Could you check a few things on this model? Use its own coordinates, in mm. A direction names the side the tool comes from. Give positions to 0.01 mm unless a question says otherwise; leave off trailing zeros. Loops run counter-clockwise (first coordinate to the right, second up) from the corner with the lowest first, then second, coordinate; pieces in that order, holes last. Notation, with made-up numbers: M 11,44 L 70,44 A14 ccw 70,51 Z; hole C 26,-20.75 d2. An arc over 180 degrees is marked long. Use CSV: the item, a comma, the result in double quotes.
```python
from build123d import *

# Parameters (mm, degrees)
F1_DEPTH = 12.7
F3_DEPTH = 12.7
F4_W     = 12.7
F4_H     = 38.1
F5_DEPTH = 12.7
F6_R     = 6.35
F7_DEPTH = 25.4
F8_R     = 6.34999


# Not quite as in the source:
# - a fillet or chamfer is up to 0.001 mm smaller than in the source, because OpenCascade refuses the exact size


with BuildPart() as f1:
    # F0 (on Top) → F1 (new body)
    with BuildSketch(Plane.XY):
        with BuildLine():
            ThreePointArc((29.6785237075, -38.1), (48.7285237075, -19.05), (29.6785237075, 0))
            Line((29.6785237075, 0), (-21.1214762925, 0))
            Line((-21.1214762925, 0), (-21.1214762925, -38.1))
            Line((-21.1214762925, -38.1), (29.6785237075, -38.1))
        make_face()
    extrude(amount=F1_DEPTH)

    # F2 (on Front) → F3 (join)
    with BuildSketch(Plane.XZ):
        with BuildLine():
            Line((-21.1026167169, 19.05), (-21.1026167169, 10.3077341521))
            Line((-21.1026167169, 10.3077341521), (4.2973832831, 10.3077341521))
            Line((4.2973832831, 10.3077341521), (4.2973832831, 19.05))
            ThreePointArc((4.2973832831, 19.05), (-8.4026167169, 31.75), (-21.1026167169, 19.05))
        make_face()
    extrude(amount=F3_DEPTH)

    # F4 (on face) → F5 (join)
    with BuildSketch(Plane.XY):
        with Locations((-14.7714762925, -19.05)):
            Rectangle(F4_W, F4_H)
    extrude(amount=-F5_DEPTH)

    # F6 (on face) → F7 (cut)
    with BuildSketch(Plane.XY.offset(12.7)):
        with Locations((29.6785237075, -19.05)):
            Circle(F6_R)
    extrude(amount=-F7_DEPTH, mode=Mode.SUBTRACT)

    # F8 (radius 6.35 in the source; OpenCascade refuses exactly that, so slightly less here)
    f8_edges = [f1.edges().sort_by_distance(p)[0] for p in [
        (4.297383, -6.35, 12.7),
    ]]
    fillet(f8_edges, radius=F8_R)


solid = f1.part
```
1. I want a section at B-B, the plane z = 3. List the corners of the cut face in (x, y) for me, then the cut area to 3 significant figures.
Outcome:
outline,"M -21.12,-38.1 L 29.68,-38.1 A19.05 ccw 29.68,0 L -21.12,0 Z; hole C 29.68,-19.05 d12.7"
area,"2,380 mm2"
2. I'm going to push flat-ended pins straight in: pin 1 Ø7 at (y, z) = (-4, 16.5) entering from -X; pin 2 Ø2 at (x, y) = (0.5, -26.5) entering from -Z; pin 3 Ø5 at (y, z) = (-6.5, -7.5) entering from +X. Where does each tip first touch, or does it pass through?
Outcome:
pin 1,"x = -21.1"
pin 2,"z = 0"
pin 3,"x = -8.42"
3. I want a section at A-A, the plane y = -19.05. List the corners of the cut face in (x, z) for me.
Outcome:
outline,"M -21.12,-12.7 L -8.42,-12.7 L -8.42,0 L 23.33,0 L 23.33,12.7 L -21.12,12.7 Z; M 36.03,0 L 48.73,0 L 48.73,12.7 L 36.03,12.7 Z"
4. If we mould it in two halves opening along Y, with no side actions, what happens to faces 1 (the face through (6.21, -6.44, 14.51)), 2 (the face through (24.639, -22.914, 6.439)), 3 (the face through (-2, -38.1, 3))? For each: +Y half, -Y half, draft (parallel to the pull), parting line (faces both ways), or undercut.
Outcome:
face 1,"draft"
face 2,"undercut"
face 3,"-Y half"
5. Please list where these lines run through material, in increasing order: line 1 (X direction, y = -19, z = 7); line 2 (Z direction, x = 19.5, y = -15.5); line 3 (Z direction, x = -9, y = -32.5).
Outcome:
line 1,"-21.12 to 23.33, 36.03 to 48.73"
line 2,"0 to 12.7"
line 3,"-12.7 to 12.7"
6. Which directions (+Z, -Z, +X, -X, +Y, -Y) give clear straight access to the entire face, cutting with the end or side of a thin tool? Please do faces 4 (the face through (-8.421, -19, -6)), 5 (the face through (48.724, -19.469, 6.261)), 6 (the face through (-9, -12.7, 22)).
Outcome:
face 4,"-Z, +X, +Y, -Y"
face 5,"+Z, -Z, +X"
face 6,"+Z, +X, -X, -Y"
7. I want a section at C-C, the plane x = 32. List the corners of the cut face in (y, z) for me, then the cut area to 3 significant figures.
Outcome:
outline,"M -37.96,0 L -24.96,0 L -24.96,12.7 L -37.96,12.7 Z; M -13.14,0 L -0.14,0 L -0.14,12.7 L -13.14,12.7 Z"
area,"330 mm2"
